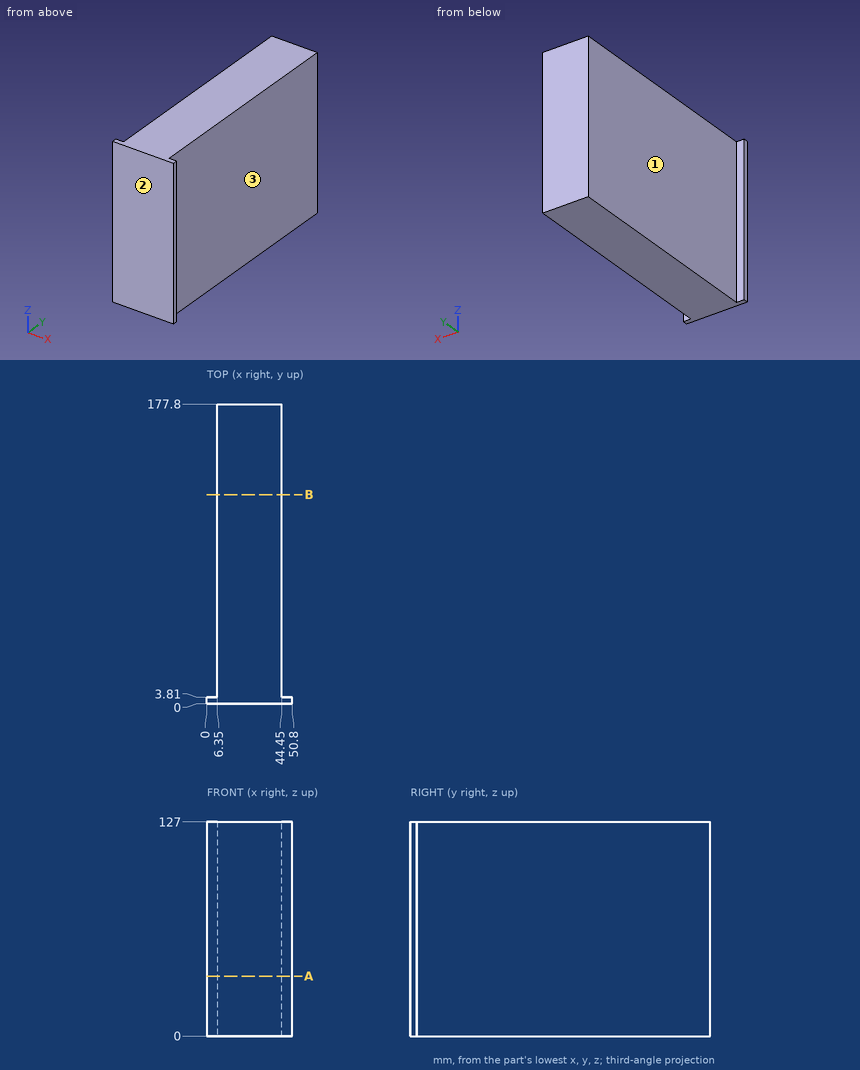
Can you work these out from the drawing? Everything is in mm from the part's minimum corner. A direction names the side the tool comes from. Round coordinates to 2 decimals unless told otherwise and drop trailing zeros. Write each loop counter-clockwise with the first axis right and the second up, starting at its lowest first coordinate (ties: lowest second). Pieces come first, ordered by that corner, then holes. Notation, with made-up numbers: (67.5, -12.75) - (108.5, -12.75) arc R21 cw to (108.5, 15.25) - close; hole circle Ø10 at (24.5, -27.5). An arc over 180 degrees is marked (long way). Use a Markdown table: item, result.
Q1. I want a section at B-B (y = 124). List the corners of the cut face in (x, z) for me.
Output values:
| item | result |
|---|---|
| outline | (6.35, 0) - (44.45, 0) - (44.45, 127) - (6.35, 127) - close |
Q2. For the marked faces 1, 2 and 3, which set-ups out of +Z, -Z, +X, -X, +Y, -Y let a thin tool reach every point of the face, with its end or its side?
Output values:
| item | result |
|---|---|
| face 1 | +Z, -Z, -X, +Y |
| face 2 | +Z, -Z, +X, -X, -Y |
| face 3 | +Z, -Z, +X, +Y |
Q3. For pin 1 (3 mm diameter, centred on y = 22, z = 99.5, fed in from -X); pin 2 (1 mm diameter, centred on y = 137, z = 37, fed in from +X); pin 3 (1.5 mm diameter, centred on x = 26, z = 76, fed in from -Y); pin 4 (1.9 mm diameter, centred on x = 48, z = 80.5, fed in from +Y), each with a flat end and sliding along its axis, tell me the tip position at first contact or that it passes through.
Output values:
| item | result |
|---|---|
| pin 1 | x = 6.35 |
| pin 2 | x = 44.45 |
| pin 3 | y = 0 |
| pin 4 | y = 3.81 |
Q4. Please list where these lines run through material, in increasing order: L1, parallel to X at y = 114.5, z = 85.5; L2, parallel to Y at x = 45, z = 16.5.
Output values:
| item | result |
|---|---|
| L1 | 6.35 to 44.45 |
| L2 | 0 to 3.81 |
Q5. I want a section at A-A (z = 35.5). List the corners of the cut face in (x, y) for me, plus the area to 3 significant figures.
Output values:
| item | result |
|---|---|
| outline | (0, 0) - (50.8, 0) - (50.8, 3.81) - (44.45, 3.81) - (44.45, 177.8) - (6.35, 177.8) - (6.35, 3.81) - (0, 3.81) - close |
| area | 6,820 mm2 |
